Verification items for the finished model (mm, model axes). Round coordinates to 2 decimals unless told otherwise and drop trailing zeros. Loops run counter-clockwise (first coordinate to the right, second up) from the corner with the lowest first, then second, coordinate; pieces in that order, holes last. Notation, with made-up numbers: (56, -3) -> (60, -3) arc R9 cw to (60, 4) -> close; hole circle Ø1 at (-13, 24). An arc over 180 degrees is marked (long way). Write item = value, one per line.
```python
from build123d import *

# Parameters (mm, degrees)
F2_R = 2.872773
F3_R = 0.969826
F4_R = 5.08


with BuildPart() as f1:
    # F0 (on Top) → F1 (revolve)
    with BuildSketch(Plane.XY):
        Polygon((125.30574, 4.5), (-34.69426, 4.5), (-34.69426, 0), (141.30574, 0), (141.30574, 1), align=None)
    revolve(axis=Axis((0.009605, 0, 0), (1, 0, 0)))

    # F2
    f2_edges = [f1.edges().sort_by_distance(p)[0] for p in [
        (-34.69426, -4.5, 0),
    ]]
    fillet(f2_edges, radius=F2_R)

    # F3
    f3_edges = [f1.edges().sort_by_distance(p)[0] for p in [
        (141.30574, -1, 0),
    ]]
    fillet(f3_edges, radius=F3_R)

    # F4
    f4_edges = [f1.edges().sort_by_distance(p)[0] for p in [
        (125.30574, -4.5, 0),
    ]]
    fillet(f4_edges, radius=F4_R)


solid = f1.part
```
(1) Sectioned sample at A-A, the plane x = 23. Record the cut outline in (y, z).
Filled sheet:
outline = circle Ø9 at (0, 0)
(2) Go/stop test with flat-tipped pins: pin 1 Ø1.5 at (x, y) = (42, -1.5) entering from +Z; pin 2 Ø1 at (y, z) = (2, 3.5) entering from -X; pin 3 Ø2 at (x, y) = (4, -1.5) entering from -Z. Record where each tip stops, or that it passes through.
Filled sheet:
pin_1 = 4.44
pin_2 = -33.97
pin_3 = -4.47
(3) Material ranges on probe 1 along Z at (x, y) = (2.5, 0.5); probe 2 along Z at (x, y) = (25, 1), recorded low to high. Write a range as from..to.
Filled sheet:
probe_1 = -4.47..4.47
probe_2 = -4.39..4.39
